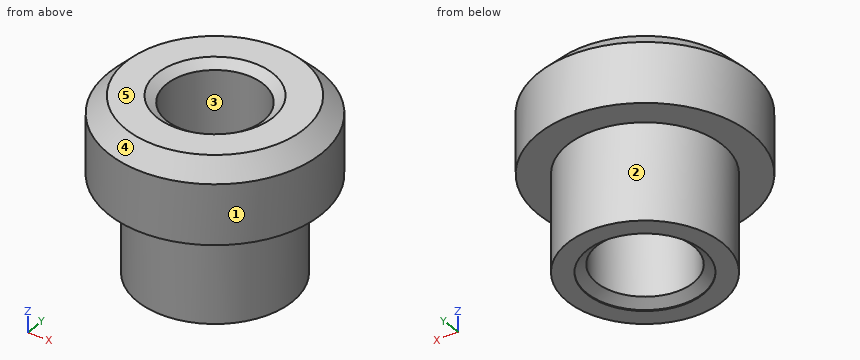
```python
from build123d import *

# Parameters (mm, degrees)
BASENUTSKE_R       = 2.75
BASENUTSKE_R_2     = 1.25
BASENUT_DEPTH      = 4.5
CHAMFER1_SIZE      = 0.45
SKETCH1_OUTSIDE_W  = 9.298
SKETCH1_OUTSIDE_H  = 9.298
SKETCH1_OUTSIDE_R  = 2
CUT_EXTRUDE1_DEPTH = 2.5


with BuildPart() as part:
    # BaseNutSke → BaseNut (new body)
    with BuildSketch(Plane.XY):
        Circle(BASENUTSKE_R)
        Circle(BASENUTSKE_R_2, mode=Mode.SUBTRACT)
    extrude(amount=-BASENUT_DEPTH)

    # EndChSke (on Right Plane) → EndChamfer (revolve, cut)
    with BuildSketch(Plane(origin=(0, 0, 0), x_dir=(0, 0, -1), z_dir=(1, 0, 0)), mode=Mode.PRIVATE) as endchamfer_sk:
        Polygon((4.4746, 1.5), (4.282042927, 1.225), (4.5254, 1.225), (4.5254, 1.5), align=None)
        Polygon((-0.0508, 1.5), (0, 1.5), (0.192557073, 1.225), (-0.0508, 1.225), align=None)
    revolve(endchamfer_sk.sketch.rotate(Axis((0, 0, -25.037505729), (0, 0, -1)), 90), axis=Axis((0, 0, -25.037505729), (0, 0, -1)), mode=Mode.SUBTRACT)

    # Chamfer1
    chamfer1_edges = [part.edges().sort_by_distance(p)[0] for p in [
        (-2.75, 0, 0),
    ]]
    chamfer(chamfer1_edges, length=CHAMFER1_SIZE)

    # Sketch1 outside → Cut-Extrude1 (cut)
    with BuildSketch(Plane(origin=(0, 0, -4.5), x_dir=(-1, 0, 0), z_dir=(0, 0, -1))):
        Rectangle(SKETCH1_OUTSIDE_W, SKETCH1_OUTSIDE_H)
        Circle(SKETCH1_OUTSIDE_R, mode=Mode.SUBTRACT)
    extrude(amount=-CUT_EXTRUDE1_DEPTH, mode=Mode.SUBTRACT)


solid = part.part
```
Work out the finished part from the listing and answer in its coordinate system (mm). Face numbers are marked on the shaded views. A direction names the side the tool comes from. Give positions to 0.01 mm unless a question says otherwise; leave off trailing zeros. Loops run counter-clockwise (first coordinate to the right, second up) from the corner with the lowest first, then second, coordinate; pieces in that order, holes last. Notation, with made-up numbers: (86.25, 2) -> (100.25, 2) arc R25 cw to (100.25, 21) -> close; hole circle Ø7 at (49, -32). An arc over 180 degrees is marked (long way). Write item = value, one per line. Start each with the question number.
(1) The mould has two halves that part along X. Classify the marked faces 3, 4 and 5: +X half, -X half, draft (parallel to the pull), parting line (faces both ways), or undercut.
(2) Find section D-D on z = -3.15. Give the vertices of the cut face in (x, y), and give its area (3 significant figures).
(3) Find the intervals of material crossed by probe 1 along Y at (x, z) = (0, -1.6); probe 2 along Y at (x, z) = (0, -2.5); probe 3 along X at (y, z) = (-0.75, -0.9), in increasing order. Write a range as from..to.
(4) Find section C-C on z = -0.3. Give the vertices of the cut face in (x, y), and give its area (3 significant figures).
(5) Which of the six approach directions +Z, -Z, +X, -X, +Y, -Y give full straight-line access (tool end or side, diameter ignored) to the marked faces 1 and 2?
(6) Given pin 1 Ø3 at (x, y) = (0.5, 0) entering from -Z, flat-ended and moving along its own axis, determine where the tip first touches the part or whether it passes through.
From the geometry:
q1.face_3 = undercut
q1.face_4 = parting line
q1.face_5 = draft
q2.outline = circle Ø4 at (0, 0); hole circle Ø2.5 at (0, 0)
q2.area = 7.66 mm^2
q3.probe_1 = -2.75..-1.25, 1.25..2.75
q3.probe_2 = -2..-1.25, 1.25..2
q3.probe_3 = -2.65..-1, 1..2.65
q4.outline = circle Ø5.2 at (0, 0); hole circle Ø2.5 at (0, 0)
q4.area = 16.3 mm^2
q5.face_1 = +Z, -Z
q5.face_2 = -Z
q6.pin_1 = -4.5
